Geometry: see drawing. Coordinates: mm, zero at the bounding-box minimum. A direction names the side the tool comes from. Round coordinates to 2 decimals unless told otherwise and drop trailing zeros. Write each loop counter-clockwise with the first axis right and the second up, starting at its lowest first coordinate (ties: lowest second). Pieces come first, ordered by that corner, then holes. Notation, with made-up numbers: (20, 55) -> (53, 55) arc R26 cw to (53, 92) -> close; hole circle Ø8 at (31, 81). An arc over 180 degrees is marked (long way). Use CSV: the item, a comma, the result in double quotes.
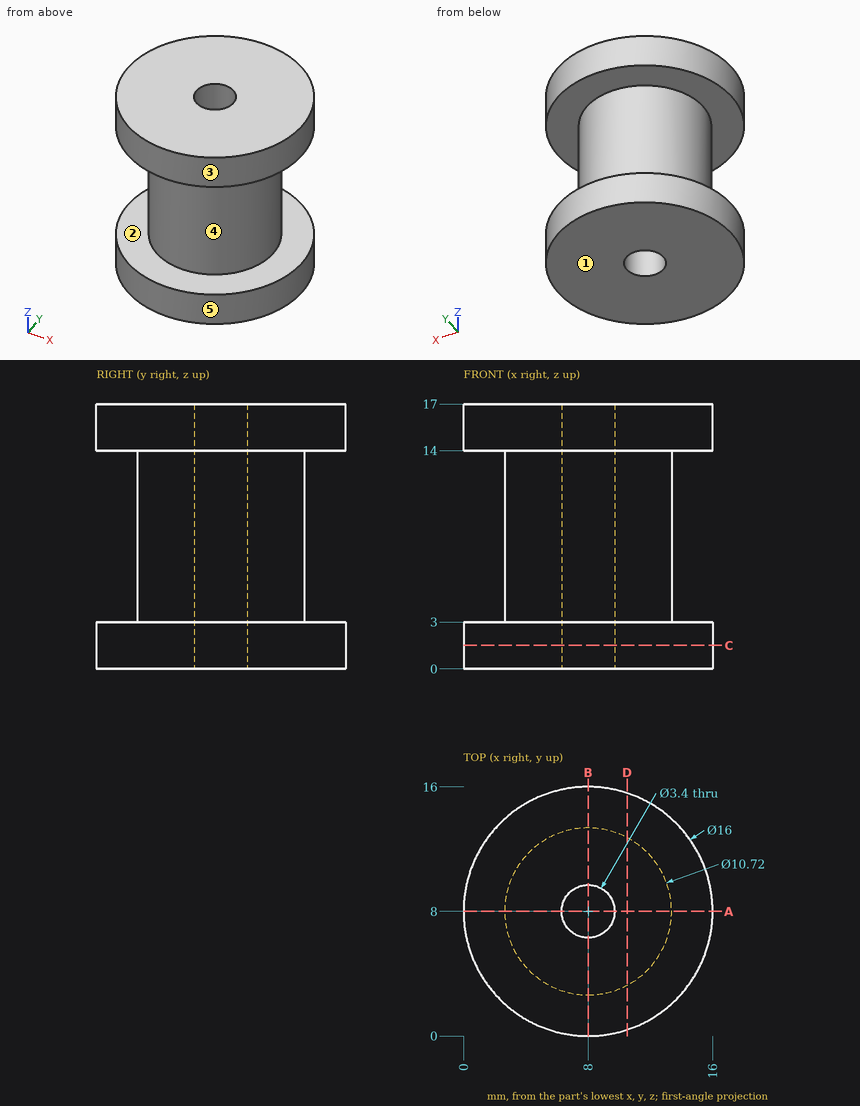
Item 1: First-contact query: pin 1 Ø6 at (x, z) = (5.5, 2) entering from -Y; pin 2 Ø1 at (y, z) = (3, 2) entering from +X; pin 3 Ø3 at (x, z) = (4.5, 6.5) entering from -Y; pin 4 Ø2 at (x, z) = (5, 4.5) entering from +Y. Flat tips, straight axial feed; report the tip coordinate or a pass-through.
Worked answers:
pin 1,"stops at y = 0"
pin 2,"stops at x = 14.61"
pin 3,"stops at y = 3.03"
pin 4,"stops at y = 12.97"
Item 2: Pull-direction query (Z, two-part tool) for the marked faces 1, 2 and 3; classes: +Z half, -Z half, draft (parallel to the pull), parting line (faces both ways), or undercut.
Worked answers:
face 1,"-Z half"
face 2,"undercut"
face 3,"draft"
Item 3: Section query C-C on z = 1.5. Return the cut outline in (x, y), plus the area to 3 significant figures.
Worked answers:
outline,"circle Ø16 at (8, 8); hole circle Ø3.4 at (8, 8)"
area,"192 mm²"
Item 4: Line query: line 1 (X direction, y = 8, z = 4.75); line 2 (Z direction, x = 14.5, y = 8.25); line 3 (Y direction, x = 7.75, z = 10.5). Output: solid intervals per line, ascending.
Worked answers:
line 1,"x = 2.64 to 6.3, 9.7 to 13.36"
line 2,"z = 0 to 3, 14 to 17"
line 3,"y = 2.65 to 6.32, 9.68 to 13.35"
Item 5: Set-up query: the marked faces 4 and 5. Return all of +Z, -Z, +X, -X, +Y, -Y with unobstructed straight access to the full face (end or side cutting, diameter ignored); none if empty.
Worked answers:
face 4,"none"
face 5,"+Z, -Z"
Item 6: Section query A-A on y = 8. Return the cut outline in (x, z).
Worked answers:
outline,"(0, 0) -> (6.3, 0) -> (6.3, 17) -> (0, 17) -> (0, 14) -> (2.64, 14) -> (2.64, 3) -> (0, 3) -> close; (9.7, 0) -> (16, 0) -> (16, 3) -> (13.36, 3) -> (13.36, 14) -> (16, 14) -> (16, 17) -> (9.7, 17) -> close"
Item 7: Section query D-D on x = 10.5. Return the cut outline in (y, z).
Worked answers:
outline,"(0.4, 0) -> (15.6, 0) -> (15.6, 3) -> (12.74, 3) -> (12.74, 14) -> (15.6, 14) -> (15.6, 17) -> (0.4, 17) -> (0.4, 14) -> (3.26, 14) -> (3.26, 3) -> (0.4, 3) -> close"
